Part model, mm, in its own coordinate system. A direction names the side the tool comes from. Give positions to 0.01 mm unless a question says otherwise; leave off trailing zeros. Order: outer loops, then holes, each group sorted by start corner. A loop starts at its lowest first (then second) coordinate and runs counter-clockwise, first axis right, second up. Notation, with made-up numbers: (54.25, -26.75) - (104.25, -26.75) arc R24 cw to (104.25, 0.25) - close; hole circle Ø9 at (60.25, -7). An arc over 180 degrees is marked (long way). Use one line per item in the form item = value. Start each with the question number.
1. Pin check, flat tips, straight feed: P1, Ø12, axis at x = -2.5, z = 1, coming from the +Y side; P2, Ø1, axis at x = 13.5, z = 0.5, coming from the +Y side; P3, Ø3.5, axis at x = -13.45, z = 6.2, coming from the +Y side; P4, Ø5, axis at x = -2, z = -6, coming from the -Y side. Stop position of each tip, or through.
2. Band-saw the part on A-A, the plane x = -13.45. List the corners of the cut face in (y, z).
3. Band-saw the part on C-C, the plane x = 4. List the corners of the cut face in (y, z).
4. Pull direction X, two halves, no side cores. Call faces 1 (the face through (11.6, -0.59, 6.14)), 2 (the face through (0, -5, 12.4)), 3 (the face through (-3.09, 15.69, -9.05)): +X half, -X half, draft (parallel to the pull), parting line (faces both ways), or undercut.
5. Band-saw the part on D-D, the plane y = 13. List the corners of the cut face in (x, z), plus the area to 3 significant figures.
6. Drill centre lines: line 1 (Z direction, x = -13.45, y = -0.3); line 2 (X direction, y = -4.5, z = 7.5); line 3 (Z direction, x = -2.75, y = 2.5). Where is each one in solid material? Low to high.
7. Band-saw the part on B-B, the plane y = -4. List the corners of the cut face in (x, z), plus the area to 3 significant figures.
8. Tool access for faces 4 (the face through (-3, 15.25, 5)), 5 (the face through (-11.5, 0.05, 5)), 6 (the face through (11.5, 0.05, 5)), 7 (the face through (0, -5, 0)): list every direction of +Z, -Z, +X, -X, +Y, -Y with a clear straight run to the whole face (end or side of a thin tool).
from build123d import *

# Parameters (mm, degrees)
BOSS_EXTRUDE1_DEPTH     = 12.4
CUT_EXTRUDE1_DEPTH      = 1.2
CUT_EXTRUDE2_DEPTH      = 3
SKETCH3_R               = 3.95
TURNBASE_DEPTH          = 7.9
BOSS_EXTRUDE3_DEPTH     = 2.7
CUT_EXTRUDE3_DEPTH      = 26.394586037
CUT_EXTRUDE3_DEPTH_BACK = 26.394586037
SKETCH6_W               = 7.25
SKETCH6_H               = 1.2
SKETCH6_W_2             = 9.95
SKETCH7_R               = 1
CUT_EXTRUDE4_DEPTH      = 38.994374584


with BuildPart() as part:
    # Sketch1 → Boss-Extrude1 (new body)
    with BuildSketch(Plane.XY):
        Polygon((-11.35, -1.25), (-11.35, -16.25), (11.35, -16.25), (11.35, -1.25), (14.85, -1.25), (14.85, 1.25), (11.35, 1.25), (11.35, 5.85), (-11.35, 5.85), (-11.35, 1.25), (-14.85, 1.25), (-14.85, -1.25), align=None)
    extrude(amount=BOSS_EXTRUDE1_DEPTH)

    # Sketch2 → Cut-Extrude1 (cut)
    with BuildSketch(Plane(origin=(0, 1.25, 0), x_dir=(1, 0, 0), z_dir=(0, 1, 0))):
        with BuildLine():
            Line((14.85, -1.3), (11.35, -1.3))
            Line((11.35, -1.3), (11.35, -11.1))
            Line((11.35, -11.1), (14.85, -11.1))
            Line((14.85, -11.1), (14.85, -7.409338662))
            ThreePointArc((14.85, -7.409338662), (11.6, -6.2), (14.85, -4.990661338))
            Line((14.85, -4.990661338), (14.85, -1.3))
        make_face()
    cut_extrude1 = extrude(amount=-CUT_EXTRUDE1_DEPTH, mode=Mode.SUBTRACT)

    # Sketch2_3 → Cut-Extrude2 (cut)
    with BuildSketch(Plane(origin=(0, 1.25, 0), x_dir=(1, 0, 0), z_dir=(0, 1, 0))):
        with BuildLine():
            Line((14.85, -7.409338662), (14.85, -4.990661338))
            ThreePointArc((14.85, -4.990661338), (11.6, -6.2), (14.85, -7.409338662))
        make_face()
    cut_extrude2 = extrude(amount=-CUT_EXTRUDE2_DEPTH, mode=Mode.SUBTRACT)

    # Mirror1: Cut-Extrude1, Cut-Extrude2 across plane
    add(cut_extrude1.mirror(Plane(origin=(0, 0, 0), x_dir=(0, 0, 1), z_dir=(1, 0, 0))), mode=Mode.SUBTRACT)
    add(cut_extrude2.mirror(Plane(origin=(0, 0, 0), x_dir=(0, 0, 1), z_dir=(1, 0, 0))), mode=Mode.SUBTRACT)

    # Sketch3 → TurnBase (add)
    with BuildSketch(Plane(origin=(0, 5.85, 0), x_dir=(1, 0, 0), z_dir=(0, 1, 0))):
        with Locations(Location((-3.15, -6.2, 0), (0, 0, 270))):
            Circle(SKETCH3_R)
    extrude(amount=TURNBASE_DEPTH)

    # Sketch4 → Boss-Extrude3 (add)
    with BuildSketch(Plane(origin=(0, 13.75, 0), x_dir=(1, 0, 0), z_dir=(0, 1, 0))):
        with BuildLine():
            Line((-5.988763946, 6.452822581), (-7.084427224, -5.849596774))
            ThreePointArc((-7.084427224, -5.849596774), (-3.15, -10.15), (0.784427224, -5.849596774))
            Line((0.784427224, -5.849596774), (-0.311236054, 6.452822581))
            ThreePointArc((-0.311236054, 6.452822581), (-3.15, 9.05), (-5.988763946, 6.452822581))
        make_face()
    extrude(amount=BOSS_EXTRUDE3_DEPTH)

    # Sketch6 → Cut-Extrude3 (cut, two sides: drawn at the far end of the back side and taken through both)
    with BuildSketch(Plane(origin=(0, 0, 0), x_dir=(0, 0, -1), z_dir=(1, 0, 0)).offset(-CUT_EXTRUDE3_DEPTH_BACK)):
        with Locations((5.425, 14.35)):
            Rectangle(SKETCH6_W, SKETCH6_H)
        with Locations((-5.175, 15.85)):
            Rectangle(SKETCH6_W_2, SKETCH6_H)
    extrude(amount=CUT_EXTRUDE3_DEPTH + CUT_EXTRUDE3_DEPTH_BACK, mode=Mode.SUBTRACT)

    # Sketch7 → Cut-Extrude4 (cut, through all)
    with BuildSketch(Plane(origin=(0, 16.45, 0), x_dir=(1, 0, 0), z_dir=(0, 1, 0))):
        with Locations(Location((-3.15, 6.2, 0), (0, 0, 270))):
            Circle(SKETCH7_R)
    extrude(amount=-CUT_EXTRUDE4_DEPTH, mode=Mode.SUBTRACT)


solid = part.part
From the geometry:
q1.P1 = 16.45
q1.P2 = 1.25
q1.P3 = through
q1.P4 = 14.95
q2.outline = (-1.25, 0) - (1.25, 0) - (1.25, 1.3) - (0.05, 1.3) - (0.05, 4.35) - (-1.25, 4.35) - close; (-1.25, 8.05) - (0.05, 8.05) - (0.05, 11.1) - (1.25, 11.1) - (1.25, 12.4) - (-1.25, 12.4) - close
q3.outline = (-16.25, 0) - (5.85, 0) - (5.85, 12.4) - (-16.25, 12.4) - close
q4.face_1 = undercut
q4.face_2 = draft
q4.face_3 = parting line
q5.outline = circle Ø7.9 at (-3.15, 6.2)
q5.area = 49.0 mm²
q6.line_1 = 0 to 4.35, 8.05 to 12.4
q6.line_2 = -11.35 to 11.35
q6.line_3 = 0 to 12.4
q7.outline = (-11.35, 0) - (11.35, 0) - (11.35, 12.4) - (-11.35, 12.4) - close
q7.area = 281 mm²
q8.face_4 = +Z, +X, -X, +Y
q8.face_5 = -X, +Y
q8.face_6 = +X, +Y
q8.face_7 = -Z, +X, -X, -Y
